Part print with two shaded views. Sizes in mm from the minimum x, y, z corner. A direction names the side the tool comes from. Round coordinates to 2 decimals unless told otherwise and drop trailing zeros. Loops run counter-clockwise (first coordinate to the right, second up) from the corner with the lowest first, then second, coordinate; pieces in that order, holes last. Notation, with made-up numbers: (-30.5, 5) -> (18.5, 5) arc R13 cw to (18.5, 15) -> close; hole circle Ø8 at (87, 78.5). An arc over 180 degrees is marked (long way). Use a Markdown table: item, result. Add a question column.
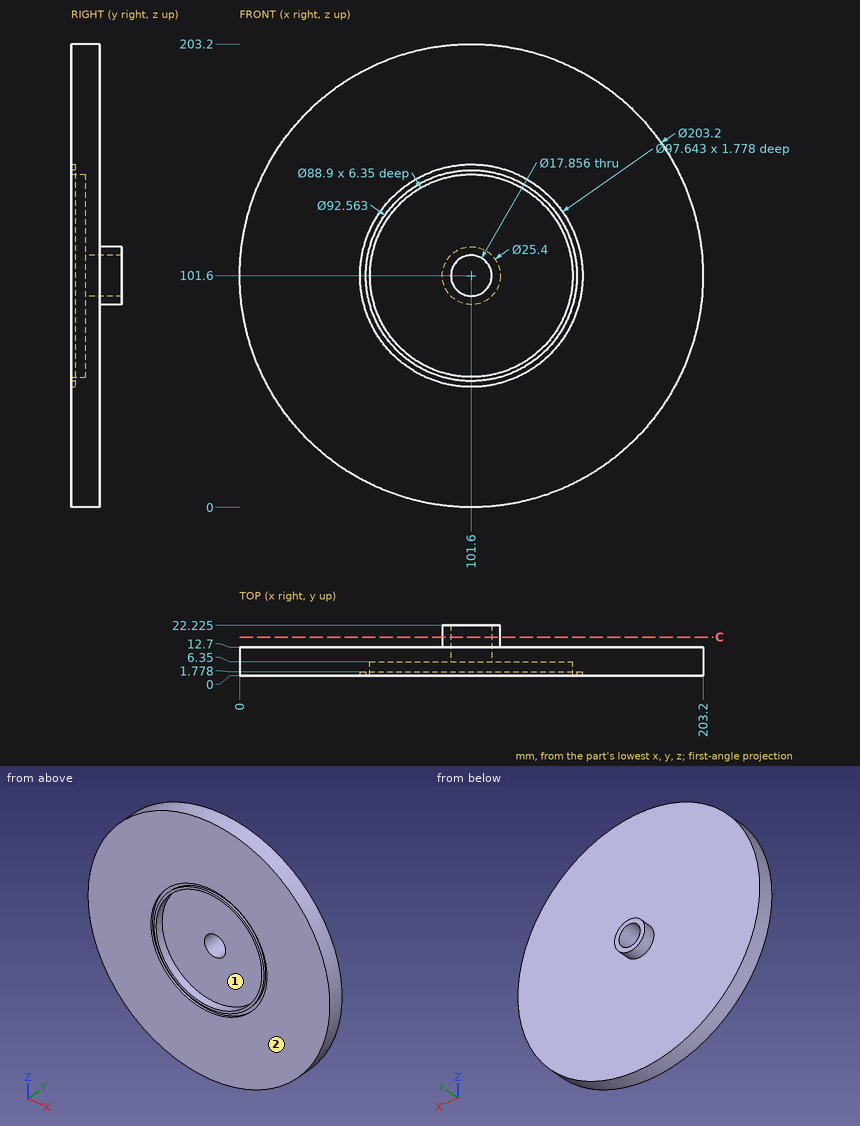
1) Tool access for the marked faces 1 and 2: list every direction of +Z, -Z, +X, -X, +Y, -Y with a clear straight run to the whole face (end or side of a thin tool).
2) Wall check: probe 1 along Z at (x, y) = (101.6, 13.5); probe 2 along Z at (x, y) = (101.6, 4.25). Give the ranges that are in metal, low to high. Write a range as from..to.
3) Pin check, flat tips, straight feed: pin 1 Ø2 at (y, z) = (8.5, 111.5) entering from -X; pin 2 Ø10 at (y, z) = (13.5, 73) entering from +X (1 decimal); pin 3 Ø8 at (x, z) = (92.5, 90) entering from -Y. Stop position of each tip, or through.
4) Cut at C-C on y = 17. Write the cut outline in (x, z), and give its area (3 significant figures).
Established:
| question | item | result |
|---|---|---|
| 1 | face 1 | -Y |
| 1 | face 2 | +Z, -Z, +X, -X, -Y |
| 2 | probe 1 | z = 88.9..92.67, 110.53..114.3 |
| 2 | probe 2 | z = 0..57.15, 146.05..203.2 |
| 3 | pin 1 | stops at x = 0.39 |
| 3 | pin 2 | stops at x = 200.4 |
| 3 | pin 3 | stops at y = 6.35 |
| 4 | outline | circle Ø25.4 at (101.6, 101.6); hole circle Ø17.86 at (101.6, 101.6) |
| 4 | area | 256 mm^2 |
